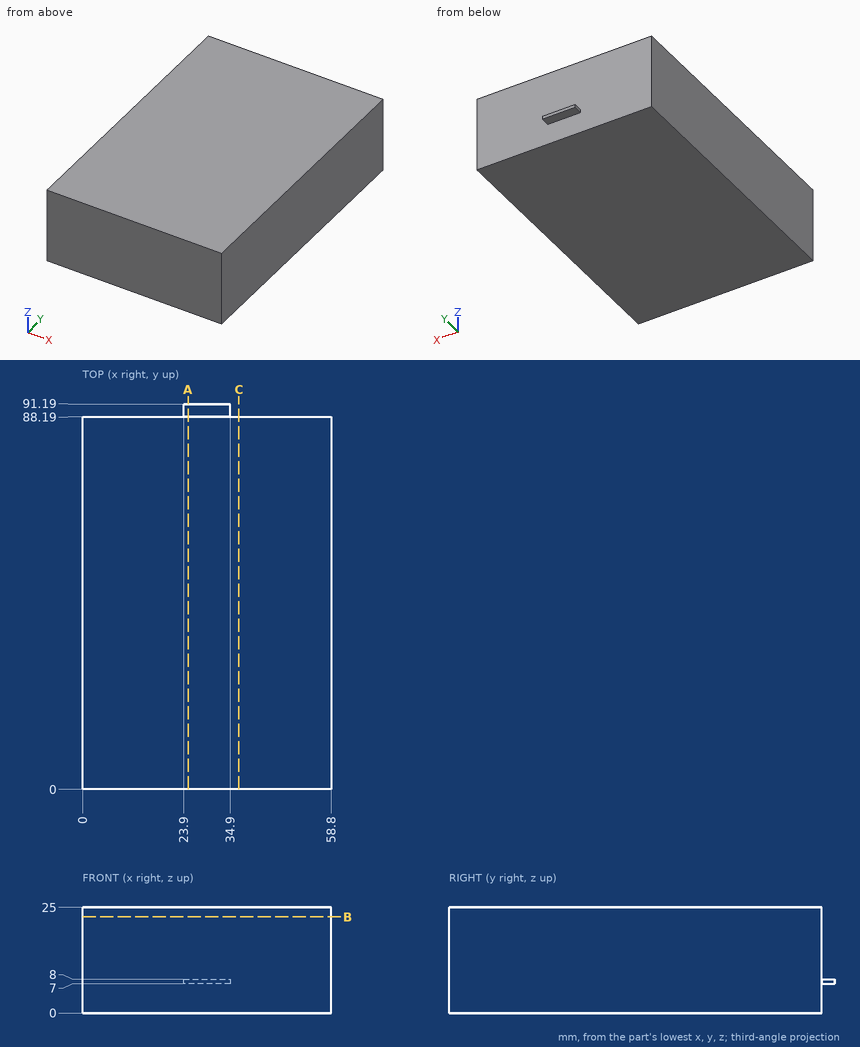
Geometry check sheet. Reference: drawing and pictorial views, mm from the part's lowest x, y, z. Round coordinates to 2 decimals unless told otherwise and drop trailing zeros. Loops run counter-clockwise (first coordinate to the right, second up) from the corner with the lowest first, then second, coordinate; pieces in that order, holes last. Notation, with made-up numbers: (-19, 5) -> (32, 5) arc R33 ccw to (32, 33) -> close; hole circle Ø8 at (-22.5, 11). An arc over 180 degrees is marked (long way). Use a Markdown table: item, result.
(1) Sectioned sample at B-B (z = 22.75). Enter the section's corners in (x, y).
Calculated:
| item | result |
|---|---|
| outline | (0, 0) -> (58.8, 0) -> (58.8, 88.19) -> (0, 88.19) -> close |
(2) Sectioned sample at A-A (x = 25). Enter the section's corners in (y, z).
Calculated:
| item | result |
|---|---|
| outline | (0, 0) -> (88.19, 0) -> (88.19, 7) -> (91.19, 7) -> (91.19, 8) -> (88.19, 8) -> (88.19, 25) -> (0, 25) -> close |
(3) Go/stop test with flat-tipped pins: P1, Ø2, axis at x = 34.5, z = 11.5, coming from the +Y side; P2, Ø0.9, axis at x = 30.5, y = 90.5, coming from the +Z side; P3, Ø1.1, axis at y = 89.5, z = 7.5, coming from the +X side. Record where each tip stops, or that it passes through.
Calculated:
| item | result |
|---|---|
| P1 | y = 88.19 |
| P2 | z = 8 |
| P3 | x = 34.9 |
(4) Sectioned sample at C-C (x = 37). Enter the section's corners in (y, z).
Calculated:
| item | result |
|---|---|
| outline | (0, 0) -> (88.19, 0) -> (88.19, 25) -> (0, 25) -> close |
(5) Scan line: probe 1 along Y at (x, z) = (37, 2). Record every from-to range of solid material in increasing order.
Calculated:
| item | result |
|---|---|
| probe 1 | 0 to 88.19 |
